Work out the finished part from the listing and answer in its coordinate system (mm). Coordinates: 2 decimals unless noted, no trailing zeros. Write each loop counter-clockwise with the first axis right and the second up, starting at its lowest first coordinate (ties: lowest second). Pieces come first, ordered by that corner, then holes. Notation, with made-up numbers: (76, 57.5) - (91, 57.5) arc R17 ccw to (91, 69.5) - close; hole circle Ø3 at (30, -16). An arc over 180 degrees is marked (long way). One line per item, written item: value.
```python
from build123d import *

# Parameters (mm, degrees)
BOSS_EXTRUDE1_START = 2.2
SKETCH1_W           = 26
SKETCH1_H           = 39
BOSS_EXTRUDE1_DEPTH = 5.5
FILLET1_R           = 2


with BuildPart() as part:
    # Sketch1 → Boss-Extrude1 (new body)
    with BuildSketch(Plane.XY.offset(BOSS_EXTRUDE1_START)):
        with Locations((0, 2.225783695)):
            Rectangle(SKETCH1_W, SKETCH1_H)
    extrude(amount=BOSS_EXTRUDE1_DEPTH)

    # Fillet1
    fillet1_edges = [part.edges().sort_by_distance(p)[0] for p in [
        (-13, 2.225783695, 7.7),
        (0, -17.274216305, 7.7),
        (13, 2.225783695, 7.7),
        (0, -17.274216305, 2.2),
        (-13, 2.225783695, 2.2),
        (0, 21.725783695, 2.2),
        (13, 2.225783695, 2.2),
        (13, -17.274216305, 4.95),
        (-13, -17.274216305, 4.95),
        (-13, 21.725783695, 4.95),
        (13, 21.725783695, 4.95),
        (0, 21.725783695, 7.7),
    ]]
    fillet(fillet1_edges, radius=FILLET1_R)


solid = part.part
```
Item 1: Consider probe 1 along Y at (x, z) = (4.25, 4.1); probe 2 along X at (y, z) = (-13, 7.2); probe 3 along X at (y, z) = (-5, 3.7). Determine where each line is inside the solid, lowest interval first.
Evaluation:
probe 1: y = -17.27 to 21.72
probe 2: x = -12.32 to 12.32
probe 3: x = -12.94 to 12.94
Item 2: Section B-B, the plane x = 11.75 is taken. Determine the outline of the cut face in (y, z), then the cut area to 3 significant figures.
Evaluation:
outline: (-17.13, 4.2) arc R1.85 ccw to (-15.27, 2.35) - (19.73, 2.35) arc R1.85 ccw to (21.58, 4.2) - (21.58, 5.7) arc R1.85 ccw to (19.73, 7.55) - (-15.27, 7.55) arc R1.85 ccw to (-17.13, 5.7) - close
area: 199 mm2
Item 3: Determine the mould class of faces 1 (the face through (-12.4, -16.7, 5)), 2 (the face through (-12.43, 2.47, 2.8)), 3 (the face through (-12.43, 21.124, 4.96)) for opening direction Y: +Y half, -Y half, draft (parallel to the pull), parting line (faces both ways), or undercut.
Evaluation:
face 1: -Y half
face 2: draft
face 3: +Y half
Item 4: Section A-A, the plane y = -3 is taken. Determine the outline of the cut face in (x, z).
Evaluation:
outline: (-13, 4.2) arc R2 ccw to (-11, 2.2) - (11, 2.2) arc R2 ccw to (13, 4.2) - (13, 5.7) arc R2 ccw to (11, 7.7) - (-11, 7.7) arc R2 ccw to (-13, 5.7) - close
